CAD build for the part. Positions are in the model's coordinates, mm. Face numbers are marked on the shaded views. Give positions to 0.01 mm unless a question says otherwise; leave off trailing zeros. Write each loop counter-clockwise with the first axis right and the second up, starting at its lowest first coordinate (ties: lowest second). Pieces come first, ordered by that corner, then holes. Notation, with made-up numbers: M 9.5,43.25 L 47.5,43.25 A9 cw 47.5,54.25 Z; hole C 38.5,71.25 d2. An arc over 180 degrees is marked long. One line per question, with ' | ' between items. Start each with the question number.
1. Wall check: L1, parallel to X at y = 112.25, z = 0 (3 decimals); L2, parallel to X at y = 112.5, z = -16; L3, parallel to X at y = 116, z = 0 (3 decimals). Give the ranges that are in metal, low to high.
2. Pull direction X, two halves, no side cores. Call the marked faces 1, 2, 3 and 4: released by +X, released by -X, zero draft, split by the parting line, or undercut.
3. Flat gauge pins, fed straight in: pin 1 (3 mm diameter, centred on y = 105.5, z = 11, fed in from +X); pin 2 (11.5 mm diameter, centred on x = 50.8, z = 0, fed in from +Y); pin 3 (1 mm diameter, centred on x = 3, z = 11, fed in from +Y). Where does each tip first touch, or does it go through?
4. Cut at A-A, the plane y = 29.5. Write the cut outline in (x, z), then the cut area to 3 significant figures.
5. Cut at B-B, the plane y = 110. Count the separate pieces of the cut face and the enclosed holes in it, then the cut area to 3 significant figures.
```python
from build123d import *
from build123d.topology import SkipClean

# Parameters (mm, degrees)
SKETCH2_R               = 10.287
BOSS_EXTRUDE1_DEPTH     = 76.2
SWEEP1_PROFILE_R        = 19.05
SKETCH10_W              = 148.15790326
SKETCH10_H              = 49.47754936
SKETCH10_R              = 10.287
CUT_EXTRUDE1_DEPTH      = 63.5
FILLET1_R               = 2.54
CUT_EXTRUDE2_DEPTH      = 63.5
CUT_EXTRUDE2_DEPTH_BACK = 63.5
SKETCH11_W              = 184.531280221
SKETCH11_H              = 85.52478337
SKETCH12_R              = 9.525
CUT_EXTRUDE3_DEPTH      = 19.05
FILLET2_R               = 1.27


with BuildPart() as part:
    # Sketch2 → Boss-Extrude1 (new body)
    with BuildSketch(Plane(origin=(0, 0, 0), x_dir=(1, 0, 0), z_dir=(0, 1, 0))):
        with Locations(Location((0, 0, 0), (0, 0, 90))):
            Circle(SKETCH2_R)
    extrude(amount=BOSS_EXTRUDE1_DEPTH)

    # Sweep1: sweep along a path in Sketch3
    with SkipClean():  # the faces are left unmerged after this step: merging them gives an invalid solid
        with BuildLine(Plane.XY) as sweep1_path:
            CenterArc((0, 127), 50.8, 0, 360)
        # Sweep1 profile (on start of the path) → Sweep1 (sweep)
        with BuildSketch(Plane(origin=(50.8, 127, 0), x_dir=(0, 0, 1), z_dir=(0, 1, 0))):
            Circle(SWEEP1_PROFILE_R)
        sweep(path=sweep1_path.line)

    # Sketch10 → Cut-Extrude1 (cut)
    with BuildSketch(Plane(origin=(0, 0, 0), x_dir=(1, 0, 0), z_dir=(0, 1, 0))):
        Rectangle(SKETCH10_W, SKETCH10_H)
        with Locations(Location((0, 0, 0), (0, 0, 90))):
            Circle(SKETCH10_R, mode=Mode.SUBTRACT)
    extrude(amount=CUT_EXTRUDE1_DEPTH, mode=Mode.SUBTRACT)

    # Fillet1
    fillet1_edges = [part.edges().sort_by_distance(p)[0] for p in [
        (9.536798122, 63.5, 13.528365302),
    ]]
    fillet(fillet1_edges, radius=FILLET1_R)

    # Sketch11 → Cut-Extrude2 (cut, two sides: drawn at the far end of the back side and taken through both)
    with BuildSketch(Plane.XY.offset(-CUT_EXTRUDE2_DEPTH_BACK)):
        with Locations((2.628650716, 169.762391685)):
            Rectangle(SKETCH11_W, SKETCH11_H)
    extrude(amount=CUT_EXTRUDE2_DEPTH + CUT_EXTRUDE2_DEPTH_BACK, mode=Mode.SUBTRACT)

    # Sketch12 → Cut-Extrude3 (cut)
    with BuildSketch(Plane(origin=(0, 127, 0), x_dir=(1, 0, 0), z_dir=(0, 1, 0))):
        with Locations(Location((50.8, 0, 0), (0, 0, 270))):
            Circle(SKETCH12_R)
        with Locations(Location((-50.8, 0, 0), (0, 0, 270))):
            Circle(SKETCH12_R)
    extrude(amount=-CUT_EXTRUDE3_DEPTH, mode=Mode.SUBTRACT)

    # Fillet2
    fillet2_edges = [part.edges().sort_by_distance(p)[0] for p in [
        (50.8, 127, -9.525),
        (-50.8, 127, -9.525),
    ]]
    fillet(fillet2_edges, radius=FILLET2_R)


solid = part.part
```
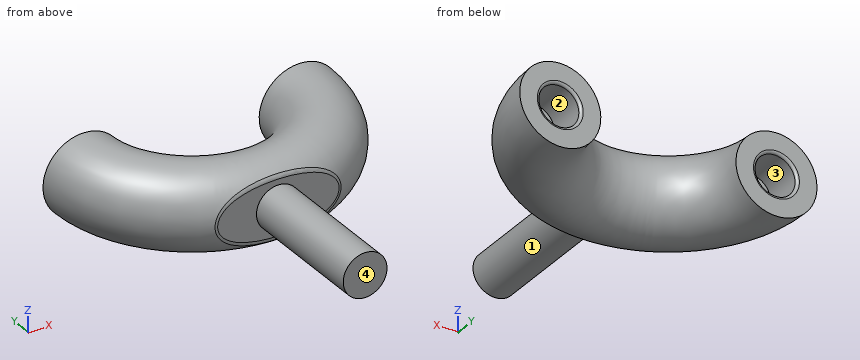
Here are the results:
1) L1: -68.275 to -60.325, -41.275 to -28.116, 28.116 to 41.275, 60.325 to 68.275 | L2: -59.4 to -37.77, 37.77 to 59.4 | L3: -68.978 to -60.325, -41.275 to -29.784, 29.784 to 41.275, 60.325 to 68.978
2) face 1: split by the parting line | face 2: undercut | face 3: undercut | face 4: zero draft
3) pin 1: x = 63.91 | pin 2: y = 107.95 | pin 3: y = 92.23
4) outline: C 0,0 d20.57 | area: 332 mm^2
5) separate pieces: 2 | enclosed holes: 2 | area: 1,870 mm^2
